Part model, mm, in its own coordinate system. Face numbers are marked on the shaded views. A direction names the side the tool comes from. Give positions to 0.01 mm unless a question says otherwise; leave off trailing zeros. Order: outer loops, then holes, each group sorted by start corner. A loop starts at its lowest first (then second) coordinate and runs counter-clockwise, first axis right, second up.
1. Slice it at D-D on x = 18.25. List the corners of the cut face in (y, z), and give its area (3 significant figures).
2. Mould opens along Y. For the marked faces 1, 2 and 3 say: +Y half, -Y half, draft (parallel to the pull), parting line (faces both ways), or undercut.
3. Which spindle directions (+Z, -Z, +X, -X, +Y, -Y) get a long thin tool onto all of the face, cutting with end or side? Do the marked faces 4 and 5. Say none if no direction does.
4. Probe line 1 (Y direction, x = 17.25, z = 0); line 2 (Y direction, x = 6.75, z = 0); line 3 (Z direction, x = 8.5, y = -2). List the from-to ranges inside material, lowest first.
5. Drop flat-ended pins along their axis: pin 1 Ø1.5 at (x, y) = (14, -22) entering from +Z; pin 2 Ø7 at (y, z) = (0, 0) entering from +X; pin 3 Ø6 at (y, z) = (1, 4.5) entering from -X; pin 4 Ø8 at (x, z) = (4.5, -2) entering from -Y. Give the stop position or say it passes through.
6. Slice it at C-C on x = 6.5. List the corners of the cut face in (y, z), and give its area (3 significant figures).
7. Slice it at A-A on y = 0. List the corners of the cut face in (x, z), and give its area (3 significant figures).
from build123d import *

# Parameters (mm, degrees)
CHAMFER_1_SIZE = 0.5
CHAMFER_2_SIZE = 0.5


with BuildPart() as part:
    # 스케치2 → 회전1 (revolve)
    with BuildSketch(Plane.XY, mode=Mode.PRIVATE) as revolve_1_sk:
        Polygon((0, 0), (0, 25), (5, 30), (20, 30), (20, 0), align=None)
    revolve(revolve_1_sk.sketch.rotate(Axis((0, 0, 0), (1, 0, 0)), 90), axis=Axis((0, 0, 0), (1, 0, 0)))

    # 스케치4 → 컷-회전1 (revolve, cut)
    with BuildSketch(Plane.XY, mode=Mode.PRIVATE) as cut_revolve_1_sk:
        Polygon((20, 7), (10, 7), (10, 4.5), (3, 4.5), (3, 10.25), (0, 10.25), (0, 0), (20, 0), align=None)
    revolve(cut_revolve_1_sk.sketch.rotate(Axis((0, 0, 0), (1, 0, 0)), 90), axis=Axis((0, 0, 0), (1, 0, 0)), mode=Mode.SUBTRACT)

    # 모따기1
    chamfer_1_edges = [part.edges().sort_by_distance(p)[0] for p in [
        (0, 0, -10.25),
        (20, 0, -7),
    ]]
    chamfer(chamfer_1_edges, length=CHAMFER_1_SIZE)

    # 모따기2
    chamfer_2_edges = [part.edges().sort_by_distance(p)[0] for p in [
        (20, 0, -30),
    ]]
    chamfer(chamfer_2_edges, length=CHAMFER_2_SIZE)


solid = part.part
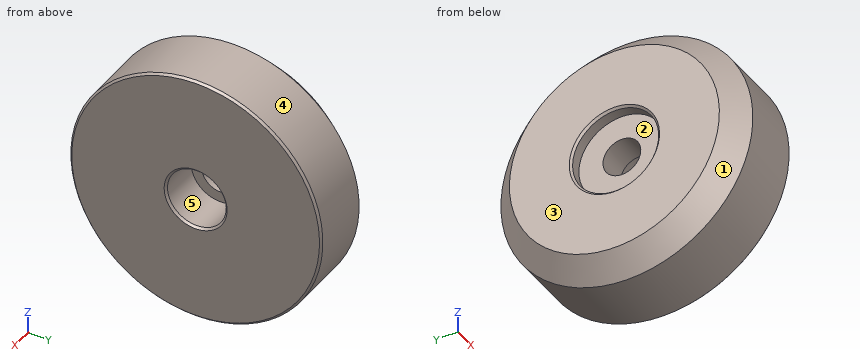
Data:
1. outline: circle Ø60 at (0, 0); hole circle Ø14 at (0, 0)
1. area: 2,670 mm2
2. face 1: parting line
2. face 2: undercut
2. face 3: draft
3. face 4: +X, -X
3. face 5: +X
4. line 1: y = -30 to -7, 7 to 30
4. line 2: y = -30 to -4.5, 4.5 to 30
4. line 3: z = -29.93 to -4.03, 4.03 to 29.93
5. pin 1: stops at z = 21.18
5. pin 2: passes through
5. pin 3: stops at x = 3
5. pin 4: stops at y = -30
6. outline: circle Ø60 at (0, 0); hole circle Ø9 at (0, 0)
6. area: 2,760 mm2
7. outline: (0, -25) - (5, -30) - (19.5, -30) - (20, -29.5) - (20, -7.5) - (19.5, -7) - (10, -7) - (10, -4.5) - (3, -4.5) - (3, -10.25) - (0.5, -10.25) - (0, -10.75) - close; (0, 10.75) - (0.5, 10.25) - (3, 10.25) - (3, 4.5) - (10, 4.5) - (10, 7) - (19.5, 7) - (20, 7.5) - (20, 29.5) - (19.5, 30) - (5, 30) - (0, 25) - close
7. area: 910 mm2
